from build123d import *

# Parameters (mm, degrees)
F0_R     = 7
F1_DEPTH = 2
F2_SIZE  = 1
F3_R     = 3
F4_DEPTH = 4


with BuildPart() as f1:
    # F0 (on Top) → F1 (new body)
    with BuildSketch(Plane.XY):
        Circle(F0_R)
    extrude(amount=F1_DEPTH)

    # F2
    f2_edges = [f1.edges().sort_by_distance(p)[0] for p in [
        (-7, 0, 2),
    ]]
    chamfer(f2_edges, length=F2_SIZE)

    # F3 (on face) → F4 (join)
    with BuildSketch(Plane(origin=(0, 0, 0), x_dir=(1, 0, 0), z_dir=(0, 0, -1))):
        Circle(F3_R)
    extrude(amount=F4_DEPTH)


solid = f1.part
Read the model definition and answer for the solid it produces. Units are mm, in the model's axes. A direction names the side the tool comes from. Round coordinates to 2 decimals unless told otherwise and drop trailing zeros. Order: outer loops, then holes, each group sorted by start corner. A loop starts at its lowest first (then second) coordinate and runs counter-clockwise, first axis right, second up. Notation, with made-up numbers: (-4, 76.5) - (35, 76.5) arc R20 cw to (35, 98.5) - close; hole circle Ø10 at (87, 61). An arc over 180 degrees is marked (long way). Use one line per item in the form item = value. Start each with the question number.
(1) For faces 1 (the face through (1, -3, 0)), 2 (the face through (6.466, -2.681, 0.493)), determine the directions among +Z, -Z, +X, -X, +Y, -Y from which every point of the face is accessible in a straight line to the end or side of a thin tool.
(2) Find the intervals of material crossed by line 1 along Z through (x, y) = (-3.5, 0); line 2 along Y through (x, z) = (3.25, 0.35); line 3 along X through (y, z) = (-6, 1.3), in increasing order. Write a range as from..to.
(3) The part is cut by section D-D (z = 0.75). Give the vertices of the cut face in (x, y).
(4) Determine the mould class of faces 3 (the face through (0, 0, -4)), 4 (the face through (-3, 0, -2)), 5 (the face through (0, 0, 2)) for opening direction Z: +Z half, -Z half, draft (parallel to the pull), parting line (faces both ways), or undercut.
(5) The part is cut by section A-A (y = 0). Give the vertices of the cut face in (x, z), then the cut area to 3 significant figures.
(6) Flat-ended cylindrical pins translate along their axes: pin 1 Ø3 at (x, y) = (-5, -1) entering from -Z; pin 2 Ø3 at (x, z) = (-5.5, 0.5) entering from +Y; pin 3 Ø3 at (x, z) = (-3, -2) entering from +Y. Find the tip coordinate at first contact, or state that the pin passes through.
(7) The part is cut by section C-C (z = -1.05). Give the vertices of the cut face in (x, y).
Checked values:
q1.face_1 = -Z
q1.face_2 = +Z, -Z
q2.line_1 = 0..2
q2.line_2 = -6.2..6.2
q2.line_3 = -2.98..2.98
q3.outline = circle Ø14 at (0, 0)
q4.face_3 = -Z half
q4.face_4 = draft
q4.face_5 = +Z half
q5.outline = (-7, 0) - (-3, 0) - (-3, -4) - (3, -4) - (3, 0) - (7, 0) - (7, 1) - (6, 2) - (-6, 2) - (-7, 1) - close
q5.area = 51.0 mm^2
q6.pin_1 = 0
q6.pin_2 = 5.74
q6.pin_3 = 2.6
q7.outline = circle Ø6 at (0, 0)
